The model under review builds one solid part; all positions refer to its coordinate system, in mm. A direction names the side the tool comes from. Round coordinates to 2 decimals unless told otherwise and drop trailing zeros. Loops run counter-clockwise (first coordinate to the right, second up) from the corner with the lowest first, then second, coordinate; pieces in that order, holes last. Notation, with made-up numbers: (12, 42.25) - (61, 42.25) arc R32 cw to (61, 76.25) - close; hole circle Ø4 at (53, 66). An arc over 180 degrees is marked (long way). Answer as CSV lines item,"result".
from build123d import *

# Parameters (mm, degrees)
SKETCH1_R           = 4
SKETCH1_R_2         = 3.999999999
SKETCH1_R_3         = 4.000000001
SKETCH1_R_4         = 4.000000002
SKETCH1_R_5         = 11.299517889
BOSS_EXTRUDE2_DEPTH = 3
SKETCH2_R           = 1.600000003
SKETCH2_R_2         = 1.599999997
CUT_EXTRUDE1_DEPTH  = 10
SKETCH3_R           = 1.6
CUT_EXTRUDE2_DEPTH  = 10
SKETCH4_W           = 50
SKETCH4_H           = 3
CUT_EXTRUDE3_DEPTH  = 167.197172059
FILLET1_R           = 1.5
FILLET2_R           = 1.5


with BuildPart() as part:
    # Sketch1 → Boss-Extrude2 (new body)
    with BuildSketch(Plane.XY):
        with BuildLine():
            Line((-112.374368671, 87.62563133), (-87.573593128, 62.824855788))
            ThreePointArc((-87.573593128, 62.824855788), (-74.567228049, 43.359454858), (-70, 20.398448917))
            Line((-70, 20.398448917), (-70, -20.398448916))
            ThreePointArc((-70, -20.398448916), (-74.567228049, -43.359454858), (-87.573593128, -62.824855787))
            Line((-87.573593128, -62.824855787), (-112.374368671, -87.625631329))
            ThreePointArc((-112.374368671, -87.625631329), (-112.374368671, -112.374368671), (-87.625631329, -112.374368671))
            Line((-87.625631329, -112.374368671), (-62.824855787, -87.573593129))
            ThreePointArc((-62.824855787, -87.573593129), (-43.359454858, -74.567228049), (-20.398448916, -70))
            Line((-20.398448916, -70), (20.398448917, -70))
            ThreePointArc((20.398448917, -70), (43.359454859, -74.567228049), (62.824855788, -87.573593129))
            Line((62.824855788, -87.573593129), (87.62563133, -112.374368671))
            ThreePointArc((87.62563133, -112.374368671), (112.374368671, -112.374368671), (112.374368671, -87.625631329))
            Line((112.374368671, -87.625631329), (87.573593129, -62.824855787))
            ThreePointArc((87.573593129, -62.824855787), (74.567228049, -43.359454858), (70, -20.398448916))
            Line((70, -20.398448916), (70, 20.398448916))
            ThreePointArc((70, 20.398448916), (74.567228049, 43.359454858), (87.573593129, 62.824855788))
            Line((87.573593129, 62.824855788), (112.374368671, 87.62563133))
            ThreePointArc((112.374368671, 87.62563133), (112.374368671, 112.374368671), (87.62563133, 112.374368671))
            Line((87.62563133, 112.374368671), (62.824855788, 87.573593129))
            ThreePointArc((62.824855788, 87.573593129), (43.359454858, 74.56722805), (20.398448916, 70))
            Line((20.398448916, 70), (-20.398448916, 70))
            ThreePointArc((-20.398448916, 70), (-43.359454858, 74.56722805), (-62.824855787, 87.573593129))
            Line((-62.824855787, 87.573593129), (-87.625631329, 112.374368671))
            ThreePointArc((-87.625631329, 112.374368671), (-112.374368671, 112.374368671), (-112.374368671, 87.62563133))
        make_face()
        with Locations((-100.000000001, 100.000000001)):
            Circle(SKETCH1_R, mode=Mode.SUBTRACT)
        with Locations((100.000000001, 100.000000001)):
            Circle(SKETCH1_R_2, mode=Mode.SUBTRACT)
        with Locations((100.000000001, -100.000000004)):
            Circle(SKETCH1_R_3, mode=Mode.SUBTRACT)
        with Locations((-100.000000001, -100.000000004)):
            Circle(SKETCH1_R_4, mode=Mode.SUBTRACT)
        with Locations((-27.108358193, -45.792037353)):
            Circle(SKETCH1_R_5, mode=Mode.SUBTRACT)
        with Locations(Location((27.108358193, -45.792037353, 0), (0, 0, 180))):
            Circle(SKETCH1_R_5, mode=Mode.SUBTRACT)
        with Locations((27.108358193, 45.792037353)):
            Circle(SKETCH1_R_5, mode=Mode.SUBTRACT)
        with Locations(Location((-27.108358193, 45.792037353, 0), (0, 0, 180))):
            Circle(SKETCH1_R_5, mode=Mode.SUBTRACT)
        with Locations(Location((-45.792037353, -27.108358193, 0), (0, 0, 180))):
            Circle(SKETCH1_R_5, mode=Mode.SUBTRACT)
        with Locations((-45.792037353, 27.108358193)):
            Circle(SKETCH1_R_5, mode=Mode.SUBTRACT)
        with Locations((45.792037353, -27.108358193)):
            Circle(SKETCH1_R_5, mode=Mode.SUBTRACT)
        with Locations(Location((45.792037353, 27.108358193, 0), (0, 0, 180))):
            Circle(SKETCH1_R_5, mode=Mode.SUBTRACT)
        with BuildLine():
            Line((11.326328369, 51.455201537), (11.326328369, 40.128873169))
            ThreePointArc((11.326328369, 40.128873169), (0, 28.8025448), (-11.326328369, 40.128873169))
            Line((-11.326328369, 40.128873169), (-11.326328369, 51.455201537))
            ThreePointArc((-11.326328369, 51.455201537), (0, 62.781529906), (11.326328369, 51.455201537))
        make_face(mode=Mode.SUBTRACT)
        with BuildLine():
            Line((11.326328369, -51.455201537), (11.326328369, -40.128873169))
            ThreePointArc((11.326328369, -40.128873169), (0, -28.8025448), (-11.326328369, -40.128873169))
            Line((-11.326328369, -40.128873169), (-11.326328369, -51.455201537))
            ThreePointArc((-11.326328369, -51.455201537), (0, -62.781529906), (11.326328369, -51.455201537))
        make_face(mode=Mode.SUBTRACT)
        with BuildLine():
            Line((51.455201537, 6.326328369), (40.128873169, 6.326328369))
            Line((40.128873169, 6.326328369), (-40.128873169, 6.326328369))
            Line((-40.128873169, 6.326328369), (-51.455201537, 6.326328369))
            ThreePointArc((-51.455201537, 6.326328369), (-57.781529906, 0), (-51.455201537, -6.326328369))
            Line((-51.455201537, -6.326328369), (-40.128873169, -6.326328369))
            Line((-40.128873169, -6.326328369), (40.128873169, -6.326328369))
            Line((40.128873169, -6.326328369), (51.455201537, -6.326328369))
            ThreePointArc((51.455201537, -6.326328369), (57.781529906, 0), (51.455201537, 6.326328369))
        make_face(mode=Mode.SUBTRACT)
    extrude(amount=BOSS_EXTRUDE2_DEPTH)

    # Sketch2 → Cut-Extrude1 (cut)
    with BuildSketch(Plane.XY.offset(3)):
        with Locations((106.717514422, 93.282485579)):
            Circle(SKETCH2_R)
        with Locations((105.65685425, 105.65685425)):
            Circle(SKETCH2_R)
        with Locations((93.282485579, 106.717514422)):
            Circle(SKETCH2_R)
        with Locations((94.343145751, 94.343145751)):
            Circle(SKETCH2_R)
        with Locations((-94.343145751, 94.343145751)):
            Circle(SKETCH2_R_2)
        with Locations((-93.282485579, 106.717514422)):
            Circle(SKETCH2_R_2)
        with Locations((-105.65685425, 105.65685425)):
            Circle(SKETCH2_R_2)
        with Locations((-106.717514422, 93.282485579)):
            Circle(SKETCH2_R_2)
        with Locations((-106.717514422, -93.282485579)):
            Circle(SKETCH2_R_2)
        with Locations((-105.65685425, -105.65685425)):
            Circle(SKETCH2_R_2)
        with Locations((-93.282485579, -106.717514422)):
            Circle(SKETCH2_R_2)
        with Locations((-94.343145751, -94.343145751)):
            Circle(SKETCH2_R_2)
        with Locations((94.343145751, -94.343145751)):
            Circle(SKETCH2_R)
        with Locations((93.282485579, -106.717514422)):
            Circle(SKETCH2_R)
        with Locations((105.65685425, -105.65685425)):
            Circle(SKETCH2_R)
        with Locations((106.717514422, -93.282485579)):
            Circle(SKETCH2_R)
    extrude(amount=-CUT_EXTRUDE1_DEPTH, mode=Mode.SUBTRACT)

    # Sketch3 → Cut-Extrude2 (cut)
    with BuildSketch(Plane(origin=(0, 0, 0), x_dir=(-1, 0, 0), z_dir=(0, 0, -1))):
        with Locations((-45, -45)):
            Circle(SKETCH3_R)
        with Locations((-45, 45)):
            Circle(SKETCH3_R)
        with Locations((45, 45)):
            Circle(SKETCH3_R)
        with Locations((45, -45)):
            Circle(SKETCH3_R)
    extrude(amount=-CUT_EXTRUDE2_DEPTH, mode=Mode.SUBTRACT)

    # Sketch4 → Cut-Extrude3 (cut, through all)
    with BuildSketch(Plane(origin=(0, 0, 0), x_dir=(-1, 0, 0), z_dir=(0, 0, -1))):
        with Locations((0, -20)):
            Rectangle(SKETCH4_W, SKETCH4_H)
        with Locations((0, 20)):
            Rectangle(SKETCH4_W, SKETCH4_H)
    extrude(amount=-CUT_EXTRUDE3_DEPTH, mode=Mode.SUBTRACT)

    # Fillet1
    fillet1_edges = [part.edges().sort_by_distance(p)[0] for p in [
        (25, 21.5, 1.5),
        (25, 18.5, 1.5),
        (-25, 18.5, 1.5),
        (-25, 21.5, 1.5),
    ]]
    fillet(fillet1_edges, radius=FILLET1_R - 0.0001)  # a hair under: the kernel refuses the full size

    # Fillet2
    fillet2_edges = [part.edges().sort_by_distance(p)[0] for p in [
        (-25, -21.5, 1.5),
        (-25, -18.5, 1.5),
        (25, -21.5, 1.5),
        (25, -18.5, 1.5),
    ]]
    fillet(fillet2_edges, radius=FILLET2_R - 0.0001)  # a hair under: the kernel refuses the full size


solid = part.part
1. Take a section at D-D (z = 2.25). State how many separate pieces and enclosed holes the cut face has, plus the area to 3 significant figures.
Numbers:
separate pieces,"1"
enclosed holes,"37"
area,"22,700 mm²"
2. Take a section at B-B (y = -2). State the section outline as (x, z) points, plus the area to 3 significant figures.
Numbers:
outline,"(-70, 0) - (-57.46, 0) - (-57.46, 3) - (-70, 3) - close; (57.46, 0) - (70, 0) - (70, 3) - (57.46, 3) - close"
area,"75.3 mm²"
3. Draft analysis for pull direction Y (two halves, no side actions). For faces 1 (the face through (-112.643, -112.099, 1.479)), 2 (the face through (43.05, -74.44, 1.48)), 3 (the face through (8, 9, 0)), state which applies: +Y half, -Y half, draft (parallel to the pull), parting line (faces both ways), or undercut.
Numbers:
face 1,"undercut"
face 2,"-Y half"
face 3,"draft"
4. Take a section at C-C (y = -100). State the section outline as (x, z) points, plus the area to 3 significant figures.
Numbers:
outline,"(-117.5, 0) - (-104, 0) - (-104, 3) - (-117.5, 3) - close; (-96, 0) - (-75.25, 0) - (-75.25, 3) - (-96, 3) - close; (75.25, 0) - (96, 0) - (96, 3) - (75.25, 3) - close; (104, 0) - (117.5, 0) - (117.5, 3) - (104, 3) - close"
area,"205 mm²"
5. Tool access review of faces 4 (the face through (-100.15, 75.4, 1.48)), 5 (the face through (0.249, 28.805, 1.479)), 6 (the face through (74.44, 43.05, 1.48)): name each direction out of +Z, -Z, +X, -X, +Y, -Y from which nothing blocks a thin tool from reaching the whole face with its end or side.
Numbers:
face 4,"+Z, -Z, -X"
face 5,"+Z, -Z"
face 6,"+Z, -Z, +X"
6. Clearance check with flat-ended pins moving along their axes: pin 1 (2.5 mm diameter, centred on x = 94.34, y = 94.34, fed in from +Z); pin 2 (0.9 mm diameter, centred on y = 44.5, z = 1, fed in from +X); pin 3 (1 mm diameter, centred on x = 3.5, z = 1, fed in from -Y); pin 4 (0.9 mm diameter, centred on y = -45, z = 1.5, fed in from -X). State where each tip first meets the part, or that it passes through.
Numbers:
pin 1,"passes through"
pin 2,"stops at x = 75.25"
pin 3,"stops at y = -70"
pin 4,"stops at x = -75.48"
7. Wall thickness on probe 1 along X at (y, z) = (32.5, 0.75); probe 2 along Y at (x, z) = (-105.5, 1); probe 3 along Y at (x, z) = (-53.5, 1.4): over which ranges is each line inside the solid? List them lowest first.
Numbers:
probe 1,"x = -71.23 to -55.72, -35.86 to -8.37, 8.37 to 35.86, 55.72 to 71.23"
probe 2,"y = -116.61 to -107.25, -104.06 to -94.32, -92.24 to -80.75, 80.75 to 92.24, 94.32 to 104.06, 107.25 to 116.61"
probe 3,"y = -79.96 to -35.37, -18.85 to -5.99, 5.99 to 18.85, 35.37 to 79.96"
8. Take a section at A-A (x = 0). State the section outline as (y, z) points.
Numbers:
outline,"(-70, 0) - (-62.78, 0) - (-62.78, 3) - (-70, 3) - close; (-28.8, 0) - (-21.5, 0) - (-21.5, 3) - (-28.8, 3) - close; (-18.5, 0) - (-6.33, 0) - (-6.33, 3) - (-18.5, 3) - close; (6.33, 0) - (18.5, 0) - (18.5, 3) - (6.33, 3) - close; (21.5, 0) - (28.8, 0) - (28.8, 3) - (21.5, 3) - close; (62.78, 0) - (70, 0) - (70, 3) - (62.78, 3) - close"
